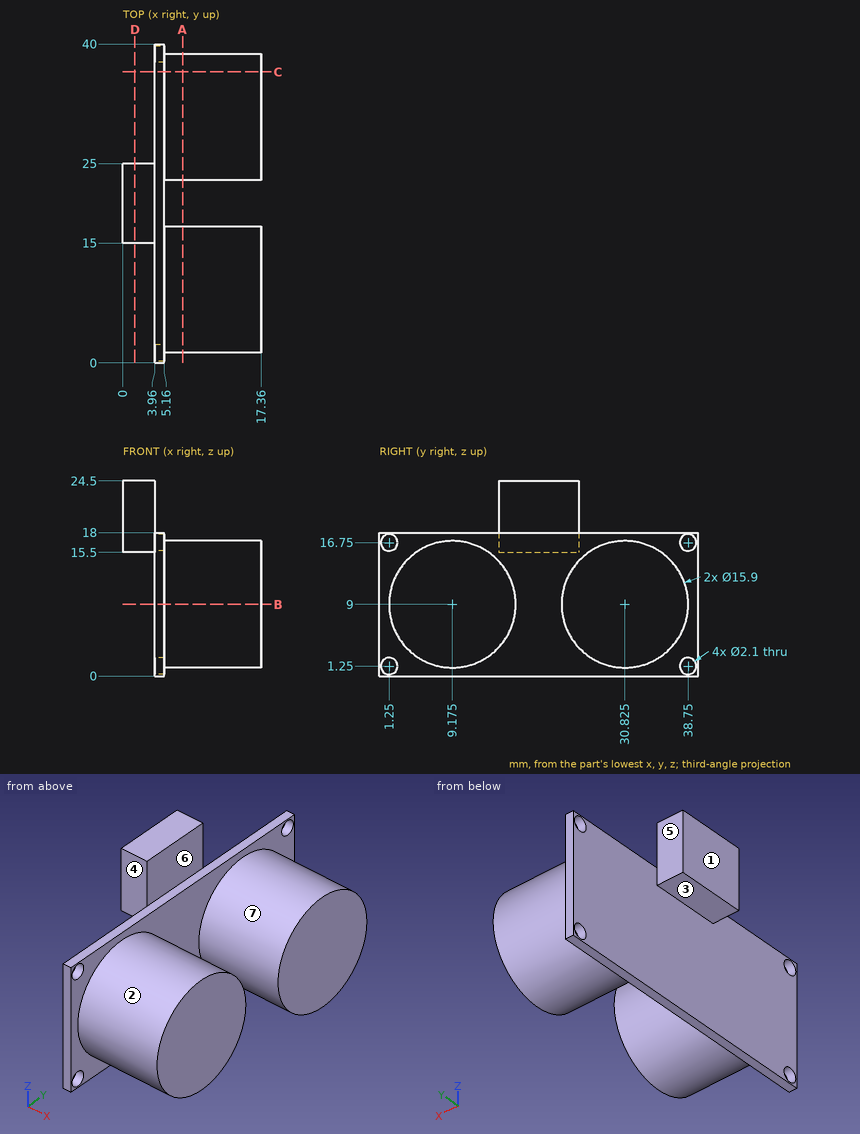
Study the drawing (mm; zero at the part's minimum x, y, z) and answer. A direction names the side the tool comes from. Round coordinates to 2 decimals unless told otherwise and drop trailing zeros. Write each loop counter-clockwise with the first axis right and the second up, starting at its lowest first coordinate (ties: lowest second). Pieces come first, ordered by that corner, then holes. Notation, with made-up numbers: (61.25, 12.25) - (76.25, 12.25) arc R18 cw to (76.25, 36.25) - close; hole circle Ø3 at (6, 68.5). An arc over 180 degrees is marked (long way). Return JSON: item names as keys, results as strings. Group by question number.
Q1. The part is cut by section B-B on z = 9. Write down the section's boundary in (x, y) (3 decimals).
Q2. For the marked faces 1, 2, 3 and 4, determine the directions among +Z, -Z, +X, -X, +Y, -Y from which every point of the face is accessible in a straight line to the end or side of a thin tool.
Q3. Find the intervals of material crossed by L1, parallel to Z at x = 4.9, y = 38.75; L2, parallel to X at y = 37.5, z = 13.25; L3, parallel to X at y = 19, z = 1, in increasing order.
Q4. The part is cut by section C-C on y = 36.5. Write down the section's boundary in (x, z), then the cut area to 3 significant figures.
Q5. Each of these flat-tipped pins is pushed along its axis until it touches: pin 1 Ø2.5 at (y, z) = (38.75, 1.25) entering from -X; pin 2 Ø2 at (x, y) = (1, 19) entering from -Z; pin 3 Ø5 at (y, z) = (18.5, 22.5) entering from +X. Where does it stop, or does it pass through?
Q6. The mould has two halves that part along Y. Classify the marked faces 5, 6 and 7: released by +Y, released by -Y, zero draft, split by the parting line, or undercut.
Q7. The part is cut by section D-D on x = 1.5. Write down the section's boundary in (y, z), then the cut area to 3 significant figures.
Q8. The part is cut by section A-A on x = 7.5. Write down the section's boundary in (y, z) (3 decimals).
Solved:
{
 "1": {"outline": "(3.96, 0) - (5.16, 0) - (5.16, 1.225) - (17.36, 1.225) - (17.36, 17.125) - (5.16, 17.125) - (5.16, 22.875) - (17.36, 22.875) - (17.36, 38.775) - (5.16, 38.775) - (5.16, 40) - (3.96, 40) - close"},
 "2": {"face 1": "+Z, -Z, -X, +Y, -Y", "face 2": "+X", "face 3": "-Z, -X, +Y, -Y", "face 4": "+Z, -Z, -X, -Y"},
 "3": {"L1": "0 to 0.2, 2.3 to 15.7, 17.8 to 18", "L2": "3.96 to 17.36", "L3": "3.96 to 5.16"},
 "4": {"outline": "(3.96, 0) - (5.16, 0) - (5.16, 3.43) - (17.36, 3.43) - (17.36, 14.57) - (5.16, 14.57) - (5.16, 18) - (3.96, 18) - close", "area": "157 mm²"},
 "5": {"pin 1": "x = 3.96", "pin 2": "z = 15.5", "pin 3": "x = 3.96"},
 "6": {"face 5": "released by +Y", "face 6": "zero draft", "face 7": "undercut"},
 "7": {"outline": "(15, 15.5) - (25, 15.5) - (25, 24.5) - (15, 24.5) - close", "area": "90.0 mm²"},
 "8": {"outline": "circle Ø15.9 at (9.175, 9); circle Ø15.9 at (30.825, 9)"}
}
